from build123d import *

# Parameters (mm, degrees)
F0_R     = 110
F0_R_2   = 23.874977
F1_DEPTH = 25.4


with BuildPart() as f1:
    # F0 (on Top) → F1 (new body)
    with BuildSketch(Plane.XY):
        Circle(F0_R)
        Polygon((8.879913, 38.905439), (35.954032, 17.314549), (35.954032, -17.314549), (8.879913, -38.905439), (-24.880962, -31.19974), (-39.905965, 0), (-24.880962, 31.19974), align=None, mode=Mode.SUBTRACT)
        with Locations((0, 79.918548)):
            Circle(F0_R_2, mode=Mode.SUBTRACT)
    extrude(amount=F1_DEPTH)


solid = f1.part
Work out the finished part from the listing and answer in its coordinate system (mm). A direction names the side the tool comes from. Give positions to 0.01 mm unless a question says otherwise; leave off trailing zeros. Order: outer loops, then holes, each group sorted by start corner. A loop starts at its lowest first (then second) coordinate and runs counter-clockwise, first axis right, second up. Notation, with made-up numbers: M 40.5,71.5 L 78.5,71.5 A15 ccw 78.5,97.5 Z; hole C 83.5,35.25 d2. An arc over 180 degrees is marked long. Return JSON: item names as keys, results as strings.
Q1. The mould has two halves that part along X. Classify faces 1 (the face through (22.23, 28.26, 12.52)), 2 (the face through (-2, -47, 0)), 3 (the face through (-32.288, -15.818, 12.522)), 4 (the face through (-23.846, -107.384, 12.522)): pulls with the +X half, pulls with the -X half, needs draft (parallel to the pull), parting line crosses it, or undercut.
Answer below:
{"face 1": "undercut", "face 2": "needs draft", "face 3": "undercut", "face 4": "parting line crosses it"}
Q2. Find section A-A, the plane y = 96. Write down the section's boundary in (x, z).
Answer below:
{"outline": "M -53.7,0 L -17.65,0 L -17.65,25.4 L -53.7,25.4 Z; M 17.65,0 L 53.7,0 L 53.7,25.4 L 17.65,25.4 Z"}
Q3. Which of the six approach directions +Z, -Z, +X, -X, +Y, -Y give full straight-line access (tool end or side, diameter ignored) to faces 5 (the face through (-2, -47, 25.4)), 6 (the face through (35.954, 0, 13))?
Answer below:
{"face 5": "+Z, +X, -X, +Y, -Y", "face 6": "+Z, -Z"}
Q4. Find section D-D, the plane z = 11.5. Write down the section's boundary in (x, y), and give its area (3 significant figures).
Answer below:
{"outline": "C 0,0 d220; hole M -39.91,0 L -24.88,-31.2 L 8.88,-38.91 L 35.95,-17.31 L 35.95,17.31 L 8.88,38.91 L -24.88,31.2 Z; hole C 0,79.92 d47.75", "area": "31,900 mm^2"}
Q5. Find section B-B, the plane x = 29.5. Write down the section's boundary in (y, z).
Answer below:
{"outline": "M -105.97,0 L -22.46,0 L -22.46,25.4 L -105.97,25.4 Z; M 22.46,0 L 105.97,0 L 105.97,25.4 L 22.46,25.4 Z"}
Q6. Find section C-C, the plane x = -12.5. Write down the section's boundary in (y, z).
Answer below:
{"outline": "M -109.29,0 L -34.03,0 L -34.03,25.4 L -109.29,25.4 Z; M 34.03,0 L 59.58,0 L 59.58,25.4 L 34.03,25.4 Z; M 100.26,0 L 109.29,0 L 109.29,25.4 L 100.26,25.4 Z"}
Q7. Each of these flat-tipped pins is pushed along its axis until it touches: pin 1 (8 mm diameter, centred on y = -19, z = 7, fed in from -X); pin 2 (6 mm diameter, centred on x = -43.5, z = 14.5, fed in from +Y); pin 3 (10 mm diameter, centred on y = 67.5, z = 9, fed in from +X). Where does it stop, or does it pass through?
Answer below:
{"pin 1": "stops at x = -108.97", "pin 2": "stops at y = 102.27", "pin 3": "stops at x = 90.52"}
Q8. Find the intervals of material crossed by line 1 along Y through (x, z) = (0, 10.5); line 2 along Y through (x, z) = (-11, 10.75); line 3 along X through (y, z) = (-5.5, 10), in increasing order. Write a range as [from, to].
Answer below:
{"line 1": "y = [-110, -36.88], [36.88, 56.04], [103.79, 110]", "line 2": "y = [-109.45, -34.37], [34.37, 58.73], [101.11, 109.45]", "line 3": "x = [-109.86, -37.26], [35.95, 109.86]"}
